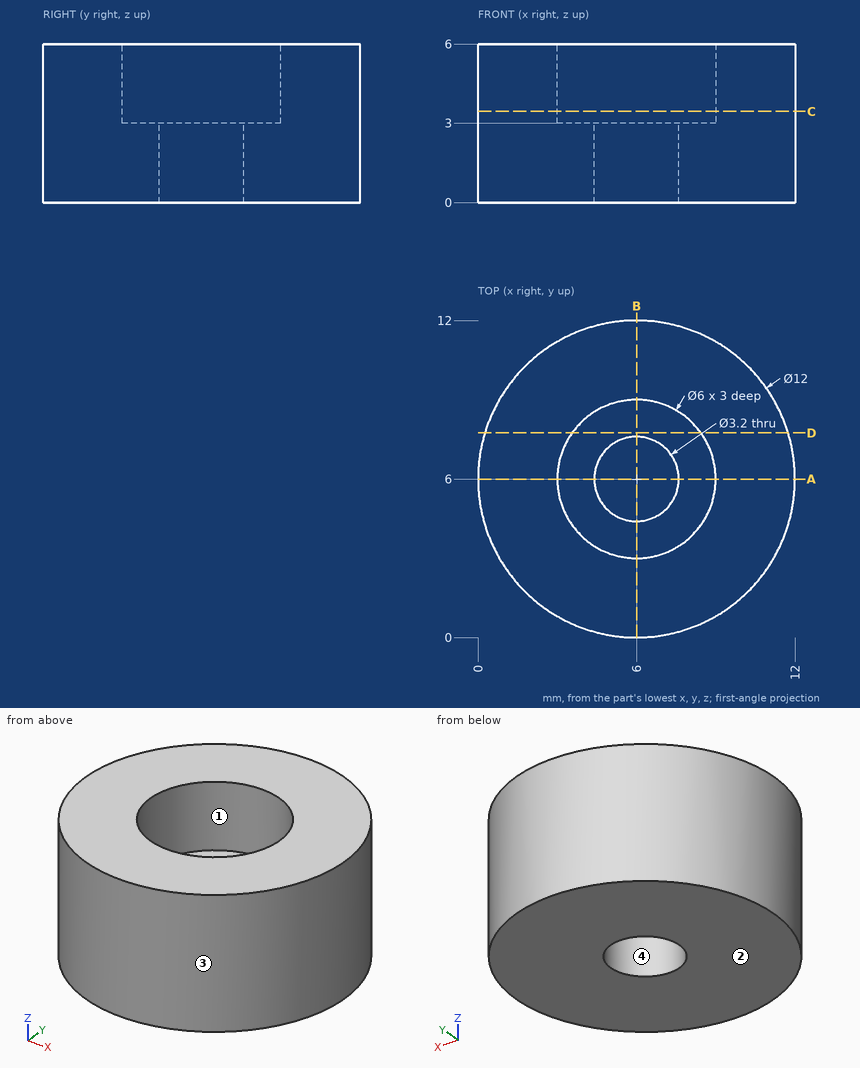
Can you work these out from the drawing? Everything is in mm from the part's minimum corner. Give positions to 0.01 mm unless a question says otherwise; leave off trailing zeros. Order: outer loops, then holes, each group sorted by start corner. A loop starts at its lowest first (then second) coordinate and runs counter-clockwise, first axis right, second up. Notation, with made-up numbers: M 4.5,47 L 31.5,47 A15 cw 31.5,68 Z; hole C -30,-18 d5. An arc over 180 degrees is marked long. Use a Markdown table: item, result. Add a question column.
Item 1: We'd pull the mould along X, two halves only. Please class the marked faces 1, 2, 3 and 4: +X half, -X half, draft (parallel to the pull), parting line (faces both ways), or undercut.
Item 2: Suppose I cut it at D-D (y = 7.75). List the corners of the cut face in (x, z) for me.
Item 3: Suppose I cut it at C-C (z = 3.45). List the corners of the cut face in (x, y) for me.
Item 4: Will these pins go through, and if not, where does the flat tip stop? pin 1 (1 mm diameter, centred on x = 1.5, z = 4, fed in from -Y); pin 2 (1 mm diameter, centred on y = 3.5, z = 3, fed in from +X).
Item 5: Suppose I cut it at A-A (y = 6). List the corners of the cut face in (x, z) for me, then the cut area to 3 significant figures.
Item 6: If I drill on L1, parallel to Y at x = 6, z = 3.9; L2, parallel to Y at x = 6, z = 1.2; L3, parallel to X at y = 6.75, z = 5.05, over which ranges is the centre line in solid material (lowest first)? Write a range as [from, to].
Answer sheet:
| question | item | result |
|---|---|---|
| 1 | face 1 | undercut |
| 1 | face 2 | draft |
| 1 | face 3 | parting line |
| 1 | face 4 | undercut |
| 2 | outline | M 0.26,0 L 11.74,0 L 11.74,6 L 8.44,6 L 8.44,3 L 3.56,3 L 3.56,6 L 0.26,6 Z |
| 3 | outline | C 6,6 d12; hole C 6,6 d6 |
| 4 | pin 1 | stops at y = 1.53 |
| 4 | pin 2 | stops at x = 11.66 |
| 5 | outline | M 0,0 L 4.4,0 L 4.4,3 L 3,3 L 3,6 L 0,6 Z; M 7.6,0 L 12,0 L 12,6 L 9,6 L 9,3 L 7.6,3 Z |
| 5 | area | 44.4 mm² |
| 6 | L1 | y = [0, 3], [9, 12] |
| 6 | L2 | y = [0, 4.4], [7.6, 12] |
| 6 | L3 | x = [0.05, 3.1], [8.9, 11.95] |
